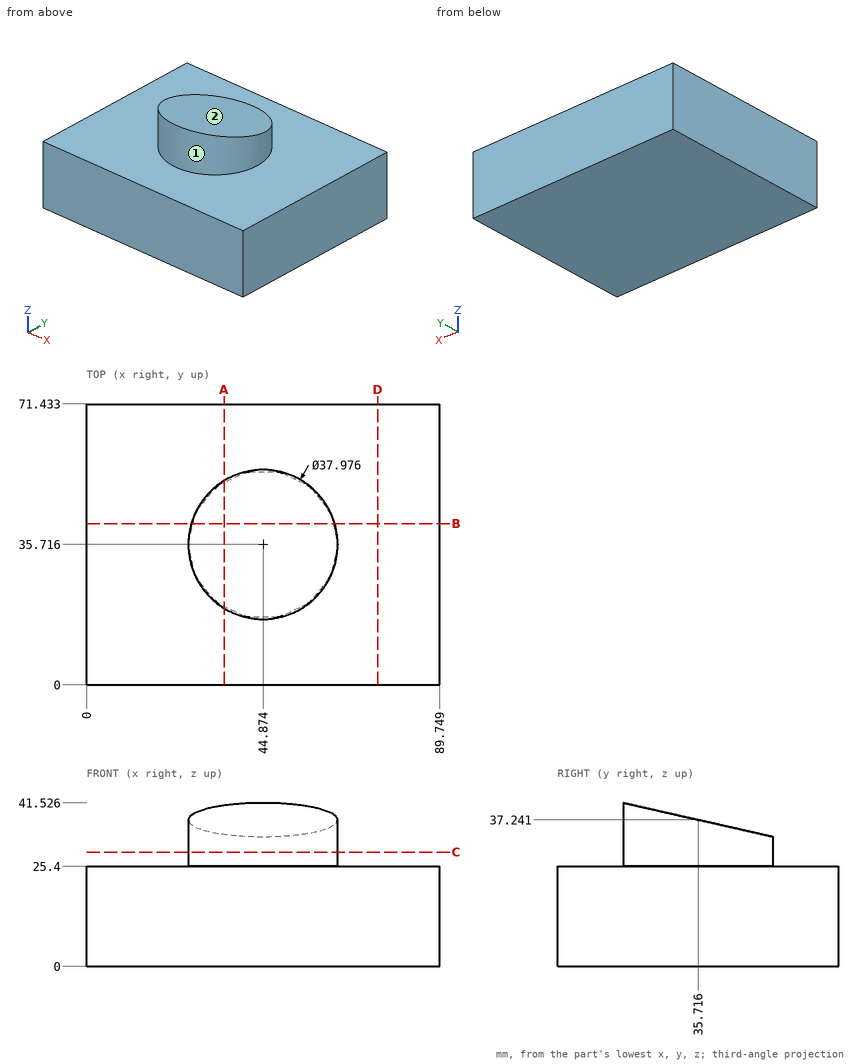
For this review, use the dimensioned drawing (mm, ordinates from the lowest corner) and the shaded views. A direction names the side the tool comes from. Give positions to 0.01 mm unless a question says otherwise; leave off trailing zeros. Order: outer loops, then holes, each group sorted by start corner. A loop starts at its lowest first (then second) coordinate and runs counter-clockwise, first axis right, second up. Notation, with made-up numbers: M -4.5,13 L 27.5,13 A20 ccw 27.5,27 Z; hole C -2,-9 d6. An arc over 180 degrees is marked long. Use one line per item in the form item = value. Start each with the question number.
Item 1: We need section C-C on z = 29. Give the boundary of the cut face in (x, y) (1 decimal), plus the area to 3 significant figures.
Item 2: To check wall thickness, follow line 1 along Z through (x, y) = (22, 30); line 2 along Z through (x, y) = (58, 23); line 3 along X through (y, z) = (39.5, 34.5). State the ranges of each line that lie inside material, in increasing order. Write a range as from..to.
Item 3: We need section D-D on x = 74. Give the boundary of the cut face in (y, z).
Item 4: We need section B-B on y = 41. Give the boundary of the cut face in (x, z).
Item 5: We need section A-A on x = 35. Give the boundary of the cut face in (y, z) (1 decimal).
Item 6: For the marked faces 1 and 2, list the 3-axis set-ups (+Z, -Z, +X, -X, +Y, -Y) from which the entire face can be reached by the end or side of a thin tool; tool diameter is ignored.
Item 7: Insertion check: pin 1 Ø5 at (y, z) = (24, 29) entering from +X (1 decimal); pin 2 Ø1 at (x, y) = (78.5, 20) entering from +Z; pin 3 Ø8 at (x, y) = (62.5, 43) entering from +Z. Each pin has a flat end and moves straight along its axis. Give the tip position at first contact, or say it passes through.
Completed:
q1.outline = C 44.9,35.7 d38
q1.area = 1,130 mm²
q2.line_1 = 0..25.4
q2.line_2 = 0..40.11
q2.line_3 = 26.27..63.48
q3.outline = M 0,0 L 71.43,0 L 71.43,25.4 L 0,25.4 Z
q4.outline = M 0,0 L 89.75,0 L 89.75,25.4 L 63.11,25.4 L 63.11,36.05 L 26.64,36.05 L 26.64,25.4 L 0,25.4 Z
q5.outline = M 0,0 L 71.4,0 L 71.4,25.4 L 51.9,25.4 L 51.9,33.6 L 19.5,40.9 L 19.5,25.4 L 0,25.4 Z
q6.face_1 = +Z
q6.face_2 = +Z, +X, -X, +Y
q7.pin_1 = 61.5
q7.pin_2 = 25.4
q7.pin_3 = 36.5
